Can you work these out from the model? Positions are in its coordinate system, mm. Give positions to 0.01 mm unless a question says otherwise; leave off trailing zeros. Order: outer loops, then holes, each group sorted by start corner. A loop starts at its lowest first (then second) coordinate and runs counter-clockwise, first axis right, second up. Notation, with made-up numbers: (61, -25.75) - (109, -25.75) arc R22 ccw to (109, -3.75) - close; hole circle Ø4 at (19, -22.5). An arc over 180 degrees is marked (long way). One line per question, with ' | ' between items.
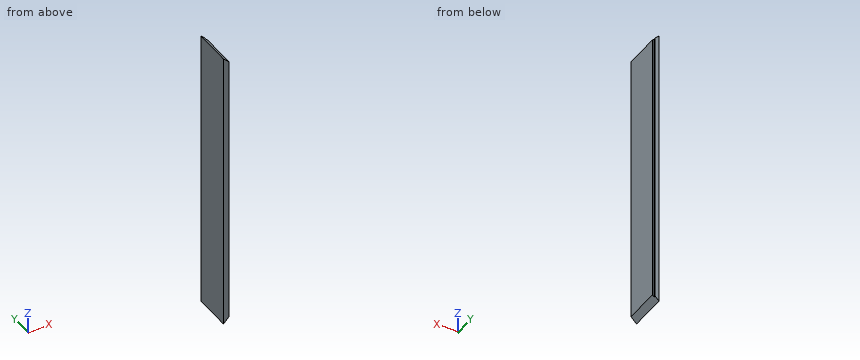
```python
from build123d import *

# Parameters (mm, degrees)
ESQUISSE1_W             = 10
ESQUISSE1_H             = 65
BOSS_EXTRU_1_DEPTH      = 520
CHANFREIN1_SIZE         = 10
ESQUISSE2_W             = 3
ESQUISSE2_H             = 3
ENL_V_MAT_EXTRU_1_DEPTH = 525.14215629


with BuildPart() as part:
    # Esquisse1 → Boss.-Extru.1 (new body)
    with BuildSketch(Plane.XY):
        with Locations((5, 32.5)):
            Rectangle(ESQUISSE1_W, ESQUISSE1_H)
    extrude(amount=BOSS_EXTRU_1_DEPTH)

    # Chanfrein1
    chanfrein1_edges = [part.edges().sort_by_distance(p)[0] for p in [
        (10, 32.5, 520),
        (10, 32.5, 0),
    ]]
    chamfer(chanfrein1_edges, length=CHANFREIN1_SIZE - 0.0001)  # a hair under: the kernel refuses the full size

    # Esquisse2 → Enlèv. mat.-Extru.1 (cut, through all)
    with BuildSketch(Plane.XY):
        with Locations((8.5, 63.5)):
            Rectangle(ESQUISSE2_W, ESQUISSE2_H)
    extrude(amount=ENL_V_MAT_EXTRU_1_DEPTH, mode=Mode.SUBTRACT)


solid = part.part
```
(1) Will these pins go through, and if not, where does the flat tip stop? pin 1 (2.5 mm diameter, centred on x = 8.5, z = 313.5, fed in from +Y); pin 2 (2 mm diameter, centred on x = 3, y = 25.5, fed in from -Z); pin 3 (0.9 mm diameter, centred on y = 63, z = 276, fed in from +X).
Answer below:
pin 1: y = 62 | pin 2: z = 2 | pin 3: x = 7
(2) Imagine slicing it at B-B (x = 4.5). List the corners of the cut face in (y, z) for me.
Answer below:
outline: (0, 4.5) - (65, 4.5) - (65, 515.5) - (0, 515.5) - close
(3) If I drill on line 1 (Y direction, x = 7.5, z = 24.5); line 2 (Z direction, x = 9.25, y = 28.5); line 3 (Z direction, x = 9.75, y = 14), over which ranges is the centre line in solid material (lowest first)?
Answer below:
line 1: 0 to 62 | line 2: 9.25 to 510.75 | line 3: 9.75 to 510.25
